Model file for the job. Use its own axes, mm. A direction names the side the tool comes from. Coordinates: 2 decimals unless noted, no trailing zeros. Order: outer loops, then holes, each group sorted by start corner. A loop starts at its lowest first (then second) coordinate and runs counter-clockwise, first axis right, second up. Notation, with made-up numbers: M 28,23 L 81,23 A13 ccw 81,34 Z; hole C 15.5,0.25 d9. An arc over 180 degrees is marked long. Return JSON: item names as keys, results as strings.
```python
from build123d import *

# Parameters (mm, degrees)
SKETCH1_W           = 406.4
SKETCH1_H           = 304.8
BOSS_EXTRUDE1_DEPTH = 15.875
SKETCH2_R           = 9.525
CUT_EXTRUDE1_DEPTH  = 16.875
CUT_EXTRUDE2_DEPTH  = 16.875


with BuildPart() as part:
    # Sketch1 → Boss-Extrude1 (new body)
    with BuildSketch(Plane.XY):
        with Locations((203.2, 152.4)):
            Rectangle(SKETCH1_W, SKETCH1_H)
    extrude(amount=BOSS_EXTRUDE1_DEPTH)

    # Sketch2 → Cut-Extrude1 (cut, through all)
    with BuildSketch(Plane.XY.offset(15.875)):
        with Locations((152.4, 228.6)):
            Circle(SKETCH2_R)
    extrude(amount=-CUT_EXTRUDE1_DEPTH, mode=Mode.SUBTRACT)

    # Sketch3 → Cut-Extrude2 (cut, through all)
    with BuildSketch(Plane.XY.offset(15.875)):
        with BuildLine():
            Line((152.4, 25.4), (0, 25.4))
            Line((0, 25.4), (0, 304.8))
            Line((0, 304.8), (355.6, 304.8))
            Line((355.6, 304.8), (355.6, 228.6))
            ThreePointArc((355.6, 228.6), (296.084097937, 84.915902063), (152.4, 25.4))
        make_face()
    extrude(amount=-CUT_EXTRUDE2_DEPTH, mode=Mode.SUBTRACT)


solid = part.part
```
Item 1: Saw through at A-A (z = 5). Write the cut outline in (x, y), and give its area (3 significant figures).
Check result:
{"outline": "M 0,0 L 406.4,0 L 406.4,304.8 L 355.6,304.8 L 355.6,228.6 A203.2 cw 152.4,25.4 L 0,25.4 Z", "area": "33,400 mm2"}
Item 2: Drop flat-ended pins along their axis: pin 1 Ø6 at (x, z) = (108, 2.5) entering from +Y; pin 2 Ø5 at (x, z) = (286.5, 4) entering from +Y; pin 3 Ø4 at (y, z) = (239, 2.5) entering from -X. Give the stop position or say it passes through.
Check result:
{"pin 1": "stops at y = 25.4", "pin 2": "stops at y = 78.17", "pin 3": "stops at x = 355.6"}
Item 3: Saw through at C-C (x = 115). Write the cut outline in (y, z) (3 decimals).
Check result:
{"outline": "M 0,0 L 25.4,0 L 25.4,15.875 L 0,15.875 Z"}
Item 4: Wall check: line 1 (X direction, y = 281.5, z = 8.5); line 2 (Y direction, x = 42, z = 1.5); line 3 (Y direction, x = 187.5, z = 11). Give the ranges that are in metal, low to high.
Check result:
{"line 1": "x = 355.6 to 406.4", "line 2": "y = 0 to 25.4", "line 3": "y = 0 to 28.45"}
Item 5: 3-axis set-ups, long thin cutter, end or side, ignore diameter. For faces 4 (the flat face through (77, 25.4, 8)), 5 (the flat face through (200, 0, 8)): which of +Z, -Z, +X, -X, +Y, -Y reach the whole face in a straight line?
Check result:
{"face 4": "+Z, -Z, -X, +Y", "face 5": "+Z, -Z, +X, -X, -Y"}
Item 6: Pull direction Z, two halves, no side cores. Call faces 1 (the flat face through (406.4, 150, 8)), 2 (the flat face through (308, 85, 15.875)), 3 (the flat face through (308, 85, 0)): +Z half, -Z half, draft (parallel to the pull), parting line (faces both ways), or undercut.
Check result:
{"face 1": "draft", "face 2": "+Z half", "face 3": "-Z half"}
Item 7: Saw through at B-B (y = 246). Write the cut outline in (x, z) (3 decimals).
Check result:
{"outline": "M 355.6,0 L 406.4,0 L 406.4,15.875 L 355.6,15.875 Z"}
